```python
from build123d import *

# Parameters (mm, degrees)
PAD_DEPTH           = 15
HOLE_D              = 6
HOLE_DEPTH          = 25
HOLE_CBORE_D        = 8
HOLE_CBORE_DEPTH    = 2
HOLE001_D           = 6
HOLE001_DEPTH       = 13
HOLE001_CBORE_D     = 8
HOLE001_CBORE_DEPTH = 2
HOLE002_D           = 6
HOLE002_DEPTH       = 13
HOLE002_CBORE_D     = 8
HOLE002_CBORE_DEPTH = 2
CHAMFER_SIZE        = 1


with BuildPart() as part:
    # Sketch → Pad (new body)
    with BuildSketch(Plane.XY):
        Polygon((0, 44), (0, 0), (44, 0), (44, 9), (38, 15), (21, 15), (15, 21), (15, 38), (9, 44), align=None)
    extrude(amount=PAD_DEPTH)

    # Hole
    with Locations(Plane.XY.offset(15)):
        with Locations((22, 7), (7, 27)):
            CounterBoreHole(HOLE_D / 2, HOLE_CBORE_D / 2, HOLE_CBORE_DEPTH, depth=HOLE_DEPTH)

    # Hole001
    with Locations(Plane.XZ):
        with Locations((6, 7), (31, 7)):
            CounterBoreHole(HOLE001_D / 2, HOLE001_CBORE_D / 2, HOLE001_CBORE_DEPTH, depth=HOLE001_DEPTH)

    # Hole002
    with Locations(Plane(origin=(0, 0, 0), x_dir=(0, -1, 0), z_dir=(-1, 0, 0))):
        with Locations((-14, 7), (-39, 7)):
            CounterBoreHole(HOLE002_D / 2, HOLE002_CBORE_D / 2, HOLE002_CBORE_DEPTH, depth=HOLE002_DEPTH)

    # Chamfer
    chamfer_edges = [part.edges().sort_by_distance(p)[0] for p in [
        (12, 41, 0),
        (15, 29.5, 0),
        (4.5, 44, 0),
        (18, 18, 0),
        (0, 22, 0),
        (29.5, 15, 0),
        (22, 0, 0),
        (41, 12, 0),
        (44, 4.5, 0),
        (4, 27, 0),
        (19, 7, 0),
    ]]
    chamfer(chamfer_edges, length=CHAMFER_SIZE)


solid = part.part
```
Build history of the part. All positions in model axes, mm. A direction names the side the tool comes from. Give positions to 0.01 mm unless a question says otherwise; leave off trailing zeros. Loops run counter-clockwise (first coordinate to the right, second up) from the corner with the lowest first, then second, coordinate; pieces in that order, holes last.
Item 1: Slice it at D-D, the plane z = 14. List the corners of the cut face in (x, y).
Answers follow:
outline: (0, 0) - (44, 0) - (44, 9) - (38, 15) - (21, 15) - (15, 21) - (15, 38) - (9, 44) - (0, 44) - close; hole circle Ø8 at (7, 27); hole circle Ø8 at (22, 7)
Item 2: Which spindle directions (+Z, -Z, +X, -X, +Y, -Y) get a long thin tool onto all of the face, cutting with end or side? Do faces 4 (the face through (6.479, 30.966, 14.014)), 5 (the face through (27, 1, 7)), 6 (the face through (7.58, 16.86, 7.9)), 7 (the face through (14.5, 29.2, 0.5)). Say none if no direction does.
Answers follow:
face 4: +Z
face 5: -Y
face 6: -X
face 7: -Z, +X, +Y
Item 3: Drill centre lines: line 1 (Y direction, x = 22, z = 5.5); line 2 (Z direction, x = 1.15, y = 39); line 3 (Y direction, x = 18, z = 8). Where is each one in solid material? Low to high.
Answers follow:
line 1: y = 0 to 4, 10 to 15
line 2: z = 0 to 3, 11 to 15
line 3: y = 0 to 18
Item 4: Pull direction Y, two halves, no side cores. Call faces 1 (the face through (12, 41, 9.5)), 2 (the face through (31, 13, 7)), 3 (the face through (18, 7, 14)): released by +Y, released by -Y, zero draft, split by the parting line, or undercut.
Answers follow:
face 1: released by +Y
face 2: released by -Y
face 3: undercut
Item 5: Flat gauge pins, fed straight in: pin 1 (1.8 mm diameter, centred on x = 30.5, z = 6.5, fed in from -Y); pin 2 (4 mm diameter, centred on x = 39.5, z = 9, fed in from +Y); pin 3 (6 mm diameter, centred on y = 25.5, z = 11, fed in from +X); pin 4 (2.5 mm diameter, centred on x = 22.5, y = 7.5, fed in from +Z). Where does each tip first touch, or does it go through?
Answers follow:
pin 1: stops at y = 13
pin 2: stops at y = 15
pin 3: stops at x = 15
pin 4: passes through
Item 6: Slice it at A-A, the plane x = 22. List the corners of the cut face in (y, z).
Answers follow:
outline: (0, 1) - (1, 0) - (3, 0) - (4, 1) - (4, 13) - (3, 13) - (3, 15) - (0, 15) - close; (10, 1) - (11, 0) - (14, 0) - (15, 1) - (15, 15) - (11, 15) - (11, 13) - (10, 13) - close
Item 7: Slice it at B-B, the plane y = 7. List the corners of the cut face in (x, z).
Answers follow:
outline: (0, 1) - (1, 0) - (18, 0) - (19, 1) - (19, 13) - (18, 13) - (18, 15) - (0, 15) - close; (25, 1) - (26, 0) - (43, 0) - (44, 1) - (44, 15) - (26, 15) - (26, 13) - (25, 13) - close; hole circle Ø6 at (6, 7); hole circle Ø6 at (31, 7)
